```python
from build123d import *

# Parameters (mm, degrees)
SKETCH2_W           = 87.535593736
SKETCH2_H           = 41.754052132
BOSS_EXTRUDE1_DEPTH = 4
SKETCH1_R           = 2.5
BOSS_EXTRUDE2_DEPTH = 55
SKETCH4_R           = 5
BOSS_EXTRUDE3_DEPTH = 2
SKETCH5_W           = 87.535593736
SKETCH5_H           = 41.754052132
SKETCH5_W_2         = 65.477303461
SKETCH5_H_2         = 31.754052132
CUT_EXTRUDE5_DEPTH  = 10
SKETCH6_R           = 5
BOSS_EXTRUDE4_DEPTH = 3
SKETCH1_3_W         = 27
SKETCH1_3_H         = 19.5
CUT_EXTRUDE1_DEPTH  = 2


with BuildPart() as part:
    # Sketch2 → Boss-Extrude1 (new body)
    with BuildSketch(Plane(origin=(0, 0, 0), x_dir=(1, 0, 0), z_dir=(0, 1, 0))):
        Rectangle(SKETCH2_W, SKETCH2_H)
    extrude(amount=-BOSS_EXTRUDE1_DEPTH)

    # Sketch1 → Boss-Extrude2 (add)
    with BuildSketch(Plane(origin=(0, 0, 0), x_dir=(1, 0, 0), z_dir=(0, 1, 0))):
        with Locations((11.961031396, 0)):
            Circle(SKETCH1_R)
        with Locations((-3.038968604, 0)):
            Circle(SKETCH1_R)
    extrude(amount=BOSS_EXTRUDE2_DEPTH)

    # Sketch4 → Boss-Extrude3 (add)
    with BuildSketch(Plane(origin=(0, 24.8, 0), x_dir=(1, 0, 0), z_dir=(0, 1, 0))):
        with Locations((11.961031396, 0)):
            Circle(SKETCH4_R)
    extrude(amount=-BOSS_EXTRUDE3_DEPTH)

    # Sketch5 → Cut-Extrude5 (cut)
    with BuildSketch(Plane(origin=(0, 0, 0), x_dir=(1, 0, 0), z_dir=(0, 1, 0))):
        Rectangle(SKETCH5_W, SKETCH5_H)
        with Locations((-6.029145138, 0)):
            Rectangle(SKETCH5_W_2, SKETCH5_H_2, mode=Mode.SUBTRACT)
    extrude(amount=-CUT_EXTRUDE5_DEPTH, mode=Mode.SUBTRACT)

    # Sketch6 → Boss-Extrude4 (add)
    with BuildSketch(Plane(origin=(0, 15.8, 0), x_dir=(1, 0, 0), z_dir=(0, 1, 0))):
        with Locations((-3.038968604, 0)):
            Circle(SKETCH6_R)
    extrude(amount=-BOSS_EXTRUDE4_DEPTH)

    # Sketch1<3> → Cut-Extrude1 (cut)
    with BuildSketch(Plane(origin=(0, 0, 0), x_dir=(1, 0, 0), z_dir=(0, 1, 0))):
        with Locations((-20.892540318, 0.894456821)):
            Rectangle(SKETCH1_3_W, SKETCH1_3_H)
    extrude(amount=-CUT_EXTRUDE1_DEPTH, mode=Mode.SUBTRACT)


solid = part.part
```
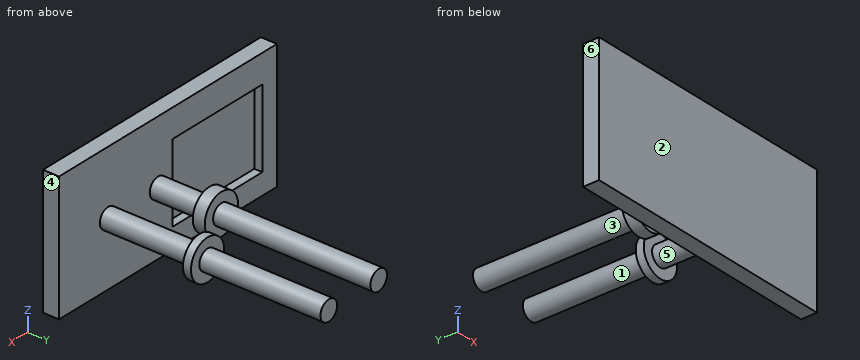
For this review, take the finished solid that the model builds, in its own axes (mm). Face numbers are marked on the shaded views. A direction names the side the tool comes from. Round coordinates to 2 decimals unless told otherwise and drop trailing zeros. Loops run counter-clockwise (first coordinate to the right, second up) from the corner with the lowest first, then second, coordinate; pieces in that order, holes last.
(1) We need section A-A (x = -22). Give the boundary of the cut face in (y, z).
Returned:
outline: (-4, -15.88) - (0, -15.88) - (0, -10.64) - (-2, -10.64) - (-2, 8.86) - (0, 8.86) - (0, 15.88) - (-4, 15.88) - close
(2) Tool access review of the marked faces 5 and 6: name each direction out of +Z, -Z, +X, -X, +Y, -Y from which nothing blocks a thin tool from reaching the whole face with its end or side.
Returned:
face 5: none
face 6: +Z, -Z, -X, +Y, -Y
(3) We need section B-B (z = 7). Give the boundary of the cut face in (x, y).
Returned:
outline: (-38.77, -4) - (26.71, -4) - (26.71, 0) - (-7.39, 0) - (-7.39, -2) - (-34.39, -2) - (-34.39, 0) - (-38.77, 0) - close
(4) Wall thickness on line 1 along X through (y, z) = (-1.5, 4); line 2 along X through (y, z) = (4, -1); line 3 along Y through (x, z) = (20, -3): over which ranges is each line inside the solid? List them lowest first.
Returned:
line 1: x = -38.77 to -34.39, -7.39 to 26.71
line 2: x = -5.33 to -0.75, 9.67 to 14.25
line 3: y = -4 to 0
(5) We need section C-C (y = 21). Give the boundary of the cut face in (x, z).
Returned:
outline: circle Ø5 at (-3.04, 0); circle Ø5 at (11.96, 0)
(6) Mouldability with a two-part tool opening along X and no side actions: class the marked faces 1, 2, 3 and 4 as released by +X, released by -X, zero draft, split by the parting line, or undercut.
Returned:
face 1: undercut
face 2: zero draft
face 3: undercut
face 4: released by +X
(7) Clearance check with flat-ended pins moving along their axes: P1, Ø10, axis at x = -16, z = 1, coming from the +Y side; P2, Ø6, axis at y = 31, z = 2.5, coming from the -X side; P3, Ø8, axis at x = 14.5, z = 6.5, coming from the +Y side. State where each tip first meets the part, or that it passes through.
Returned:
P1: stops at y = -2
P2: stops at x = -5.54
P3: stops at y = 24.8
